Geometry: final body of the model. Coordinates: model frame, mm. Give positions to 0.01 mm unless a question says otherwise; leave off trailing zeros. Write each loop counter-clockwise with the first axis right and the second up, starting at its lowest first coordinate (ties: lowest second). Pieces come first, ordered by that corner, then holes. Notation, with made-up numbers: M 13.5,64 L 66.5,64 A29 cw 66.5,85 Z; hole C -4,5 d5. An arc over 180 degrees is marked long. Use a Markdown table: item, result. Add a question column.
1) Line query: line 1 (Z direction, x = 15, y = -1.5); line 2 (Z direction, x = 17.5, y = -9.5); line 3 (X direction, y = -34, z = -63). Output: solid intervals per line, ascending.
2) Section B-B on x = 2.5. Return the cut outline in (y, z) (1 decimal), then the cut area to 3 significant figures.
3) Pin query (flat end, axial travel): pin 1 (4 mm diameter, centred on y = 1.1, z = -18.72, fed in from -X); pin 2 (3 mm diameter, centred on y = -1, z = -17, fed in from -X). Return the tip coordinate at first contact, or that it passes through.
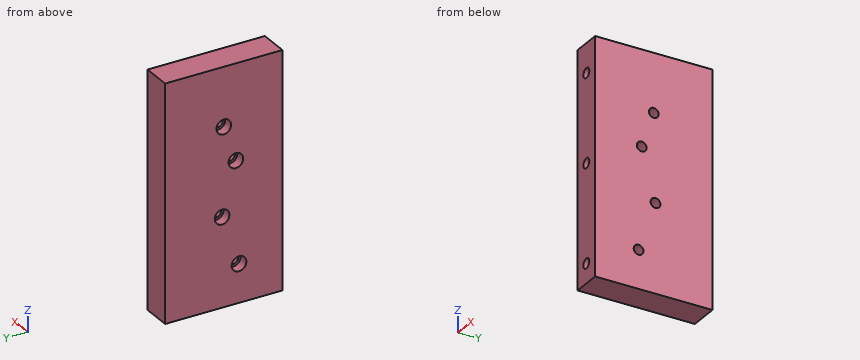
```python
from build123d import *

# Parameters (mm, degrees)
SKETCH1_R                       = 3.175
BOSS_EXTRUDE1_DEPTH             = 19.05
SKETCH2_R                       = 4.7625
CUT_EXTRUDE1_DEPTH              = 6.35
F_1_4_0_25_DIAMETER_HOLE1_D     = 6.35
F_1_4_0_25_DIAMETER_HOLE1_DEPTH = 12.7
F_1_4_0_25_DIAMETER_HOLE1_TIP   = 1.907732465


with BuildPart() as part:
    # Sketch1 → Boss-Extrude1 (new body)
    # profile 1 of 2: a face of its own
    with BuildSketch(Plane(origin=(0, 0, 0), x_dir=(0, 0, -1), z_dir=(1, 0, 0))):
        with BuildLine():
            Line((-76.2, 38.1), (-76.2, 0))
            Line((-76.2, 0), (-41.275, 0))
            ThreePointArc((-41.275, 0), (-38.1, 3.175), (-34.925, 0))
            Line((-34.925, 0), (15.74272634, 0))
            ThreePointArc((15.74272634, 0), (18.16587039, 4.221897852), (21.89753158, 1.096077429))
            ThreePointArc((21.89753158, 1.096077429), (21.848352003, 0.539416238), (21.70233682, 0))
            Line((21.70233682, 0), (76.2, 0))
            Line((76.2, 0), (76.2, 38.1))
            Line((76.2, 38.1), (-76.2, 38.1))
        make_face()
    # profile 2 of 2: a face of its own
    with BuildSketch(Plane(origin=(0, 0, 0), x_dir=(0, 0, -1), z_dir=(1, 0, 0))):
        with BuildLine():
            Line((-41.275, 0), (-76.2, 0))
            Line((-76.2, 0), (-76.2, -38.1))
            Line((-76.2, -38.1), (76.2, -38.1))
            Line((76.2, -38.1), (76.2, 0))
            Line((76.2, 0), (21.70233682, 0))
            ThreePointArc((21.70233682, 0), (18.72253158, -2.078922571), (15.74272634, 0))
            Line((15.74272634, 0), (-34.925, 0))
            ThreePointArc((-34.925, 0), (-38.1, -3.175), (-41.275, 0))
        make_face()
        with Locations(Location((-14.571224015, -7.860160654, 0), (0, 0, 180))):
            Circle(SKETCH1_R, mode=Mode.SUBTRACT)
        with Locations(Location((51.408255992, -9.873506971, 0), (0, 0, 180))):
            Circle(SKETCH1_R, mode=Mode.SUBTRACT)
    extrude(amount=BOSS_EXTRUDE1_DEPTH)

    # Sketch2 → Cut-Extrude1 (cut)
    with BuildSketch(Plane.ZY):
        with Locations((38.1, 0)):
            Circle(SKETCH2_R)
        with Locations((14.571224015, -7.860160654)):
            Circle(SKETCH2_R)
        with Locations((-18.72253158, 1.096077429)):
            Circle(SKETCH2_R)
        with Locations((-51.408255992, -9.873506971)):
            Circle(SKETCH2_R)
    extrude(amount=-CUT_EXTRUDE1_DEPTH, mode=Mode.SUBTRACT)

    # 1_4 _0.25_ Diameter Hole1
    with Locations(Plane.XZ.offset(38.1)):
        with Locations((9.525, -63.5), (9.525, 0), (9.525, 57.15)):
            Hole(F_1_4_0_25_DIAMETER_HOLE1_D / 2, depth=F_1_4_0_25_DIAMETER_HOLE1_DEPTH)
            with Locations((0, 0, -(F_1_4_0_25_DIAMETER_HOLE1_DEPTH + F_1_4_0_25_DIAMETER_HOLE1_TIP / 2))):  # 118° drill point
                Cone(0, F_1_4_0_25_DIAMETER_HOLE1_D / 2, F_1_4_0_25_DIAMETER_HOLE1_TIP, mode=Mode.SUBTRACT)


solid = part.part
```
Found:
| question | item | result |
|---|---|---|
| 1 | line 1 | -76.2 to -20.55, -16.89 to 35.3, 40.9 to 76.2 |
| 1 | line 2 | -76.2 to -54.56, -48.26 to 11.85, 17.29 to 76.2 |
| 1 | line 3 | 0 to 6.39, 12.66 to 19.05 |
| 2 | outline | M -38.1,-76.2 L 38.1,-76.2 L 38.1,76.2 L -38.1,76.2 Z; hole C -9.9,-51.4 d9.5; hole C -7.9,14.6 d9.5; hole C 0,38.1 d9.5; hole C 1.1,-18.7 d9.5 |
| 2 | area | 11,300 mm² |
| 3 | pin 1 | through |
| 3 | pin 2 | x = 6.35 |
